Can you work these out from the drawing? Everything is in mm from the part's minimum corner. A direction names the side the tool comes from. Give positions to 0.01 mm unless a question says otherwise; leave off trailing zeros. Order: outer loops, then holes, each group sorted by start corner. A loop starts at its lowest first (then second) coordinate and runs counter-clockwise, first axis right, second up. Notation, with made-up numbers: (49.5, 41) - (80.5, 41) arc R26 ccw to (80.5, 70) - close; hole circle Ø3 at (35.25, 23.25). An arc over 180 degrees is marked (long way). One line per question, with ' | ' between items.
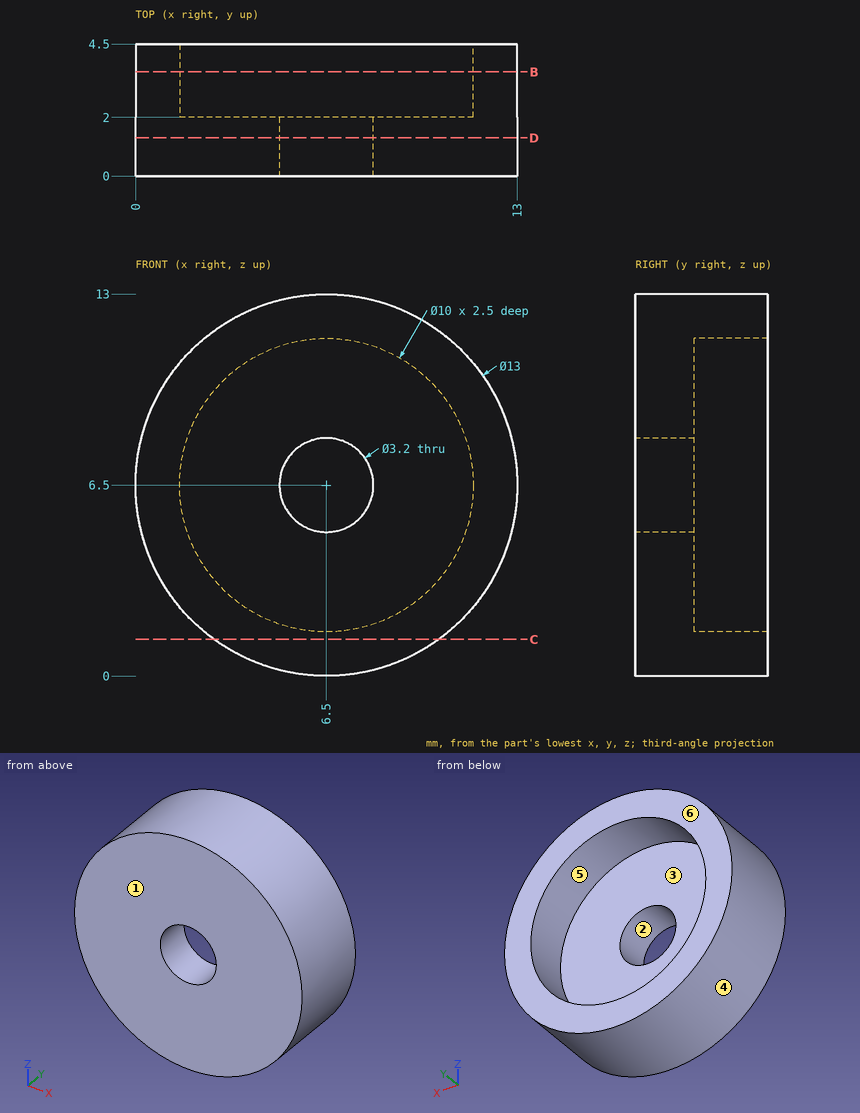
(1) On a 3-axis mill with a long thin cutter (end or side, diameter ignored), from which of +Z, -Z, +X, -X, +Y, -Y can I reach the whole of each face in a straight line? I mean the marked faces 5 and 6. Say none if no direction works.
Answer below:
face 5: +Y | face 6: +Z, -Z, +X, -X, +Y
(2) If we mould it in two halves opening along X, with no side actions, what happens to the marked faces 1, 2, 3 and 4? For each: released by +X, released by -X, zero draft, split by the parting line, or undercut.
Answer below:
face 1: zero draft | face 2: undercut | face 3: undercut | face 4: split by the parting line
(3) Imagine slicing it at D-D (y = 1.3). List the corners of the cut face in (x, z) for me, and give its area (3 significant figures).
Answer below:
outline: circle Ø13 at (6.5, 6.5); hole circle Ø3.2 at (6.5, 6.5) | area: 125 mm^2
(4) Imagine slicing it at C-C (z = 1.25). List the corners of the cut face in (x, y) for me, and give its area (3 significant figures).
Answer below:
outline: (2.67, 0) - (10.33, 0) - (10.33, 4.5) - (2.67, 4.5) - close | area: 34.5 mm^2
(5) If I drill on line 1 (X direction, y = 3.35, z = 6.5); line 2 (Z direction, x = 5.25, y = 0.4), over which ranges is the centre line in solid material (lowest first)?
Answer below:
line 1: 0 to 1.5, 11.5 to 13 | line 2: 0.12 to 5.5, 7.5 to 12.88
(6) Imagine slicing it at B-B (y = 3.55). List the corners of the cut face in (x, z) for me, and give its area (3 significant figures).
Answer below:
outline: circle Ø13 at (6.5, 6.5); hole circle Ø10 at (6.5, 6.5) | area: 54.2 mm^2
(7) Will these pins go through, and if not, where does the flat tip stop? pin 1 (2 mm diameter, centred on x = 6.5, z = 9.5, fed in from +Y); pin 2 (2.5 mm diameter, centred on x = 6.5, z = 6.5, fed in from -Y).
Answer below:
pin 1: y = 2 | pin 2: through
